```python
from build123d import *

# Parameters (mm, degrees)
CROQUIS1_W              = 28
CROQUIS1_H              = 300
SALIENTE_EXTRUIR1_DEPTH = 1.5
CROQUIS2_R              = 5
CORTAR_EXTRUIR1_DEPTH   = 151.681783902


with BuildPart() as part:
    # Croquis1 → Saliente-Extruir1 (new, symmetric)
    with BuildSketch(Plane.XY):
        Rectangle(CROQUIS1_W, CROQUIS1_H)
    extrude(amount=SALIENTE_EXTRUIR1_DEPTH, both=True)

    # Croquis2 → Cortar-Extruir1 (cut, through all)
    with BuildSketch(Plane(origin=(0, 0, -1.5), x_dir=(-1, 0, 0), z_dir=(0, 0, -1))):
        with Locations((0, 140)):
            Circle(CROQUIS2_R)
        with Locations(Location((0, -140, 0), (0, 0, 180))):
            Circle(CROQUIS2_R)
    extrude(amount=-CORTAR_EXTRUIR1_DEPTH, mode=Mode.SUBTRACT)


solid = part.part
```
Here's how the part is built. I have some questions about the finished solid (model axes, mm). Give positions to 0.01 mm unless a question says otherwise; leave off trailing zeros. Write each loop counter-clockwise with the first axis right and the second up, starting at its lowest first coordinate (ties: lowest second). Pieces come first, ordered by that corner, then holes. Notation, with made-up numbers: M 47.25,-36 L 80.25,-36 A16 ccw 80.25,-7 Z; hole C 25.25,58.5 d2. An arc over 180 degrees is marked long. Put each result on its own line as item: value. Start each with the question number.
Item 1: Will this pin go through, and if not, where does the flat tip stop? pin 1 (11.5 mm diameter, centred on x = 0, y = 140, fed in from -Z).
Item 2: I need wall thicknesses on L1, parallel to Y at x = 0, z = 0.55; L2, parallel to X at y = -140, z = -0.7; L3, parallel to Y at x = -2.25, z = -0.65. Which ranges of each line are inside material? Lowest first, please. Write a range as from..to.
Item 3: If we section it at A-A, the plane y = 140: Write out the boundary of the cut face in (x, z), then the cut area to 3 significant figures.
Item 4: If we section it at B-B, the plane x = 0: Write out the boundary of the cut face in (y, z), then the cut area to 3 significant figures.
Item 5: If we section it at C-C, the plane z = 0.75: Write out the boundary of the cut face in (x, y), then the cut area to 3 significant figures.
Item 6: Thinking about a two-plate mould opening in X: for faces 1 (the flat face through (0, 2, 1.5)), 2 (the cylindrical face through (1.08, 135.12, -0.02)), which applies, +X half, -X half, draft (parallel to the pull), parting line (faces both ways), or undercut?
Values:
1. pin 1: z = -1.5
2. L1: -150..-145, -135..135, 145..150
2. L2: -14..-5, 5..14
2. L3: -150..-144.47, -135.53..135.53, 144.47..150
3. outline: M -14,-1.5 L -5,-1.5 L -5,1.5 L -14,1.5 Z; M 5,-1.5 L 14,-1.5 L 14,1.5 L 5,1.5 Z
3. area: 54.0 mm²
4. outline: M -150,-1.5 L -145,-1.5 L -145,1.5 L -150,1.5 Z; M -135,-1.5 L 135,-1.5 L 135,1.5 L -135,1.5 Z; M 145,-1.5 L 150,-1.5 L 150,1.5 L 145,1.5 Z
4. area: 840 mm²
5. outline: M -14,-150 L 14,-150 L 14,150 L -14,150 Z; hole C 0,-140 d10; hole C 0,140 d10
5. area: 8,240 mm²
6. face 1: draft
6. face 2: undercut
